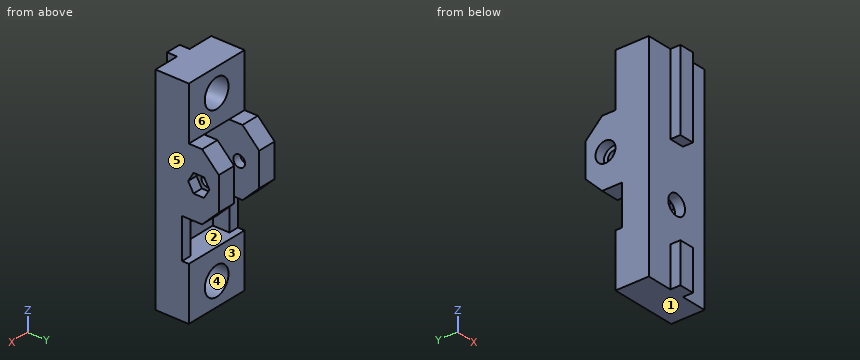
```python
from build123d import *

# Parameters (mm, degrees)
SKETCH1_W               = 20
SKETCH1_H               = 30
BOSS_EXTRUDE1_DEPTH     = 3
SKETCH2_W               = 4.5
SKETCH2_H               = 12
BOSS_EXTRUDE2_DEPTH     = 3
SKETCH3_R               = 7
SKETCH3_R_2             = 4.25
BOSS_EXTRUDE3_DEPTH     = 7
SKETCH4_R               = 4.25
BOSS_EXTRUDE4_DEPTH     = 1
CUT_EXTRUDE1_DEPTH      = 20.339079606
CUT_EXTRUDE1_DEPTH_BACK = 20.339079606
SKETCH5_R               = 3
SKETCH6_R               = 7
SKETCH6_R_2             = 4.25
BOSS_EXTRUDE6_DEPTH     = 7
SKETCH7_W               = 20
SKETCH7_H               = 3
BOSS_EXTRUDE7_DEPTH     = 19
SKETCH8_W               = 4.5
SKETCH8_H               = 3
BOSS_EXTRUDE8_DEPTH     = 12
SKETCH10_W              = 5.5
SKETCH10_H              = 20
BOSS_EXTRUDE9_DEPTH     = 16
CUT_EXTRUDE2_DEPTH      = 57.231663678
CUT_EXTRUDE2_DEPTH_BACK = 57.231663678
SKETCH11_R              = 1.75
SKETCH12_R              = 3
SKETCH12_R_2            = 1.75
CUT_EXTRUDE3_DEPTH      = 3
CUT_EXTRUDE4_START      = -3
SKETCH13_R              = 1.75
CUT_EXTRUDE4_DEPTH      = 3
CHAMFER2_SIZE           = 5
CUT_EXTRUDE5_START      = -1.5
SKETCH14_R              = 4.25
CUT_EXTRUDE5_DEPTH      = 1.5
SKETCH15_W              = 3
SKETCH15_H              = 12
BOSS_EXTRUDE10_DEPTH    = 5


with BuildPart() as part:
    # Sketch1 → Boss-Extrude1 (new body)
    with BuildSketch(Plane(origin=(0, 0, 0), x_dir=(1, 0, 0), z_dir=(0, 1, 0))):
        Rectangle(SKETCH1_W, SKETCH1_H)
    boss_extrude1 = extrude(amount=BOSS_EXTRUDE1_DEPTH)

    # Sketch2 → Boss-Extrude2 (add)
    with BuildSketch(Plane.XZ):
        with Locations((0, -9)):
            Rectangle(SKETCH2_W, SKETCH2_H)
    boss_extrude2 = extrude(amount=BOSS_EXTRUDE2_DEPTH)

    # Sketch3 → Boss-Extrude3 (add)
    with BuildSketch(Plane(origin=(0, 3, 0), x_dir=(1, 0, 0), z_dir=(0, 1, 0))):
        with Locations(Location((0, 8, 0), (0, 0, 90))):
            Circle(SKETCH3_R)
        with Locations(Location((0, 8, 0), (0, 0, 270))):
            Circle(SKETCH3_R_2, mode=Mode.SUBTRACT)
    boss_extrude3 = extrude(amount=BOSS_EXTRUDE3_DEPTH)

    # Sketch4 → Boss-Extrude4 (add)
    with BuildSketch(Plane(origin=(0, 3, 0), x_dir=(1, 0, 0), z_dir=(0, 1, 0))):
        with Locations(Location((0, 8, 0), (0, 0, 270))):
            Circle(SKETCH4_R)
    boss_extrude4 = extrude(amount=BOSS_EXTRUDE4_DEPTH)

    # Sketch5 → Cut-Extrude1 (cut, two sides: drawn at the far end of the back side and taken through both)
    with BuildSketch(Plane(origin=(0, 3, 0), x_dir=(1, 0, 0), z_dir=(0, 1, 0)).offset(-CUT_EXTRUDE1_DEPTH_BACK)):
        with Locations(Location((0, -8.5, 0), (0, 0, 90))):
            Circle(SKETCH5_R)
    extrude(amount=CUT_EXTRUDE1_DEPTH + CUT_EXTRUDE1_DEPTH_BACK, mode=Mode.SUBTRACT)

    # Sketch6 → Boss-Extrude6 (add)
    # profile 1 of 2: a face of its own
    with BuildSketch(Plane(origin=(0, 3, 0), x_dir=(1, 0, 0), z_dir=(0, 1, 0))):
        Polygon((0, 15), (-10, 15), (-10, -1), (10, -1), (10, 15), align=None)
        with BuildLine():
            ThreePointArc((7, 8), (-4.949747468, 3.050252532), (0, 15))
            ThreePointArc((0, 15), (4.949747468, 12.949747468), (7, 8))
        make_face(mode=Mode.SUBTRACT)
    # profile 2 of 2: a face of its own
    with BuildSketch(Plane(origin=(0, 3, 0), x_dir=(1, 0, 0), z_dir=(0, 1, 0))):
        with Locations((0, 8)):
            Circle(SKETCH6_R)
        with Locations(Location((0, 8, 0), (0, 0, 270))):
            Circle(SKETCH6_R_2, mode=Mode.SUBTRACT)
    boss_extrude6 = extrude(amount=BOSS_EXTRUDE6_DEPTH)

    # Sketch7 → Boss-Extrude7 (add)
    with BuildSketch(Plane.XY.offset(15)):
        with Locations((0, 1.5)):
            Rectangle(SKETCH7_W, SKETCH7_H)
    extrude(amount=BOSS_EXTRUDE7_DEPTH)

    # Mirror3: Boss-Extrude1, Boss-Extrude2, Boss-Extrude3, Boss-Extrude4, Boss-Extrude6 across plane
    add(boss_extrude1.mirror(Plane.XY.offset(17)))
    add(boss_extrude2.mirror(Plane.XY.offset(17)))
    add(boss_extrude3.mirror(Plane.XY.offset(17)))
    add(boss_extrude4.mirror(Plane.XY.offset(17)))
    add(boss_extrude6.mirror(Plane.XY.offset(17)))

    # Sketch8 → Boss-Extrude8 (add)
    with BuildSketch(Plane(origin=(0, 0, 37), x_dir=(-1, 0, 0), z_dir=(0, 0, -1))):
        with Locations((0, -1.5)):
            Rectangle(SKETCH8_W, SKETCH8_H)
    extrude(amount=BOSS_EXTRUDE8_DEPTH)

    # Sketch10 → Boss-Extrude9 (add)
    with BuildSketch(Plane(origin=(0, 3, 0), x_dir=(1, 0, 0), z_dir=(0, 1, 0))):
        with Locations((-7.25, -23)):
            Rectangle(SKETCH10_W, SKETCH10_H)
        with Locations((7.25, -23)):
            Rectangle(SKETCH10_W, SKETCH10_H)
    extrude(amount=BOSS_EXTRUDE9_DEPTH)

    # Sketch11 → Cut-Extrude2 (cut, two sides: drawn at the far end of the back side and taken through both)
    with BuildSketch(Plane.ZY.offset(10).offset(-CUT_EXTRUDE2_DEPTH_BACK)):
        with Locations((23, 13)):
            Circle(SKETCH11_R)
    extrude(amount=CUT_EXTRUDE2_DEPTH + CUT_EXTRUDE2_DEPTH_BACK, mode=Mode.SUBTRACT)

    # Sketch12 → Cut-Extrude3 (cut)
    with BuildSketch(Plane.ZY.offset(10)):
        with Locations((23, 13)):
            Circle(SKETCH12_R)
        with Locations((23, 13)):
            Circle(SKETCH12_R_2, mode=Mode.SUBTRACT)
    extrude(amount=-CUT_EXTRUDE3_DEPTH, mode=Mode.SUBTRACT)

    # Sketch13 → Cut-Extrude4 (cut)
    with BuildSketch(Plane(origin=(10, 0, 0), x_dir=(0, 0, -1), z_dir=(1, 0, 0)).offset(CUT_EXTRUDE4_START)):
        Polygon((-23, 16.175426481), (-25.75, 14.58771324), (-25.75, 11.41228676), (-23, 9.824573519), (-20.25, 11.41228676), (-20.25, 14.58771324), align=None)
        with Locations((-23, 13)):
            Circle(SKETCH13_R, mode=Mode.SUBTRACT)
    extrude(amount=CUT_EXTRUDE4_DEPTH, mode=Mode.SUBTRACT)

    # Chamfer2
    chamfer2_edges = [part.edges().sort_by_distance(p)[0] for p in [
        (-7.25, 19, 13),
        (-7.25, 19, 33),
        (7.25, 19, 13),
        (7.25, 19, 33),
    ]]
    chamfer(chamfer2_edges, length=CHAMFER2_SIZE)

    # Sketch14 → Cut-Extrude5 (cut)
    with BuildSketch(Plane(origin=(0, 4, 0), x_dir=(1, 0, 0), z_dir=(0, 1, 0)).offset(CUT_EXTRUDE5_START)):
        with Locations(Location((0, -42, 0), (0, 0, 90))):
            Circle(SKETCH14_R)
        with Locations(Location((0, 8, 0), (0, 0, 270))):
            Circle(SKETCH14_R)
    extrude(amount=CUT_EXTRUDE5_DEPTH, mode=Mode.SUBTRACT)

    # Sketch15 → Boss-Extrude10 (add)
    with BuildSketch(Plane(origin=(0, 3, 0), x_dir=(1, 0, 0), z_dir=(0, 1, 0))):
        with Locations((-8.5, -7)):
            Rectangle(SKETCH15_W, SKETCH15_H)
        with Locations((8.5, -7)):
            Rectangle(SKETCH15_W, SKETCH15_H)
    extrude(amount=BOSS_EXTRUDE10_DEPTH)


solid = part.part
```
Verification items for the finished model (mm, model axes). Face numbers are marked on the shaded views. A direction names the side the tool comes from. Give positions to 0.01 mm unless a question says otherwise; leave off trailing zeros. Loops run counter-clockwise (first coordinate to the right, second up) from the corner with the lowest first, then second, coordinate; pieces in that order, holes last.
1. Go/stop test with flat-tipped pins: pin 1 Ø1.5 at (y, z) = (-1.5, -7) entering from -X; pin 2 Ø4 at (x, z) = (3.5, 41.5) entering from +Y; pin 3 Ø4 at (y, z) = (13, 23) entering from +X; pin 4 Ø1 at (x, y) = (2.5, 14) entering from +Z. Record where each tip stops, or that it passes through.
2. Section check B-B, the plane y = 13. Enter the section's corners in (x, z), then the cut area to 3 significant figures.
3. Thickness scan on line 1 (Y direction, x = -6.1, z = 23); line 2 (X direction, y = 5, z = 17); line 3 (Z direction, x = 5.9, y = 13). Record the ranges inside material, lowest first.
4. Section check A-A, the plane z = 8.5. Enter the section's corners in (x, y), then the cut area to 3 significant figures.
5. Section check C-C, the plane x = 1. Enter the section's corners in (y, z), then the cut area to 3 significant figures.
6. Section check D-D, the plane x = 8.25. Enter the section's corners in (y, z).
7. Set-up check for the marked faces 4, 5 and 6: record each of +Z, -Z, +X, -X, +Y, -Y from which the full face is reachable in a straight line by a thin tool's end or side.
8. Mould release check, pull along Z, two halves, no side actions. Record for the marked faces 1, 2 and 3: released by +Z, released by -Z, zero draft, split by the parting line, or undercut.
Geometry says:
1. pin 1: stops at x = -2.25
1. pin 2: stops at y = 10
1. pin 3: stops at x = 7
1. pin 4: passes through
2. outline: (-10, 13) - (-4.5, 13) - (-4.5, 21.25) - (-7, 21.25) - (-7, 20) - (-10, 20) - close; (-10, 26) - (-7, 26) - (-7, 24.75) - (-4.5, 24.75) - (-4.5, 33) - (-10, 33) - close; (4.5, 13) - (10, 13) - (10, 20.25) - (7, 20.25) - (7, 21.25) - (4.5, 21.25) - close; (4.5, 24.75) - (7, 24.75) - (7, 25.75) - (10, 25.75) - (10, 33) - (4.5, 33) - close
2. area: 168 mm2
3. line 1: y = 0 to 11.25, 14.75 to 19
3. line 2: x = -10 to -4.5, 4.5 to 10
3. line 3: z = 13 to 21.25, 24.75 to 33
4. outline: (-10, 0) - (-3, 0) - (-3, 3) - (-7, 3) - (-7, 8) - (-10, 8) - close; (3, 0) - (10, 0) - (10, 8) - (7, 8) - (7, 3) - (3, 3) - close
4. area: 72.0 mm2
5. outline: (-3, -15) - (10, -15) - (10, -12.13) - (2.5, -12.13) - (2.5, -3.87) - (10, -3.87) - (10, 1) - (3, 1) - (3, 5.67) - (0, 5.67) - (0, -3) - (-3, -3) - close; (-3, 25) - (0, 25) - (0, 11.33) - (3, 11.33) - (3, 33) - (10, 33) - (10, 37.87) - (2.5, 37.87) - (2.5, 46.13) - (10, 46.13) - (10, 49) - (-3, 49) - close
5. area: 383 mm2
6. outline: (0, -15) - (10, -15) - (10, 1) - (8, 1) - (8, 13) - (14, 13) - (19, 18) - (19, 28) - (14, 33) - (10, 33) - (10, 49) - (0, 49) - close; hole (9.82, 23) - (11.41, 20.25) - (14.59, 20.25) - (16.18, 23) - (14.59, 25.75) - (11.41, 25.75) - close
7. face 4: +Y
7. face 5: +Z, -Z, +X, +Y, -Y
7. face 6: +Z, +X, -X, +Y
8. face 1: released by -Z
8. face 2: undercut
8. face 3: zero draft
